```python
from build123d import *

# Parameters (mm, degrees)
SKETCH1_R           = 6
BOSS_EXTRUDE1_DEPTH = 4


with BuildPart() as part:
    # Sketch1 → Boss-Extrude1 (new body)
    with BuildSketch(Plane(origin=(0, 0, 0), x_dir=(1, 0, 0), z_dir=(0, 1, 0))):
        Polygon((9.814954576, 0), (4.907477288, 8.5), (-4.907477288, 8.5), (-9.814954576, 0), (-4.907477288, -8.5), (4.907477288, -8.5), align=None)
        with Locations(Location((0, 0, 0), (0, 0, 270))):
            Circle(SKETCH1_R, mode=Mode.SUBTRACT)
    extrude(amount=BOSS_EXTRUDE1_DEPTH)

    # Sketch2 → Cut-Revolve1 (revolve, cut)
    with BuildSketch(Plane.XY):
        Polygon((-9.814954576, 3.422649731), (-8.814954576, 4), (-9.814954576, 4), align=None)
        Polygon((-9.814954576, 0), (-9.814954576, 0.577350269), (-8.814954576, 0), align=None)
    revolve(axis=Axis((0, 0, 0), (0, 1, 0)), mode=Mode.SUBTRACT)


solid = part.part
```
CAD build for the part. Positions are in the model's coordinates, mm. Round coordinates to 2 decimals unless told otherwise and drop trailing zeros. Order: outer loops, then holes, each group sorted by start corner. A loop starts at its lowest first (then second) coordinate and runs counter-clockwise, first axis right, second up. Notation, with made-up numbers: (-40, 57.25) - (1, 57.25) arc R23 cw to (1, 85.25) - close; hole circle Ø6 at (-2.75, 75.25). An arc over 180 degrees is marked (long way). Answer in a Markdown table with one row per item. Add a question column.
(1) Drop a flat-ended pin along its axis: pin 1 Ø1.5 at (x, y) = (-7.5, 2) entering from +Z. Give the stop position or say it passes through.
(2) Probe L1, parallel to X at y = 2.1, z = 2; L2, parallel to X at y = 0.8, z = -5.5; L3, parallel to Z at x = -2, y = 1.95. List the from-to ranges inside material, lowest first. Write a range as [from, to].
(3) Band-saw the part on D-D on x = -6.75. List the corners of the cut face in (y, z), and give its area (3 significant figures).
(4) Mould opens along X. For faces 1 (the face through (-4.515, 0.156, -7.885)), 2 (the face through (1.802, 1.972, 5.723)), 3 (the face through (-2, 4, -6)) say: +X half, -X half, draft (parallel to the pull), parting line (faces both ways), or undercut.
(5) Band-saw the part on C-C on z = -5.25. List the corners of the cut face in (x, y), and give its area (3 significant figures).
(6) Band-saw the part on B-B on y = 1. List the corners of the cut face in (x, z).
(7) Band-saw the part on A-A on x = 0. List the corners of the cut face in (y, z), and give its area (3 significant figures).
Data:
| question | item | result |
|---|---|---|
| 1 | pin 1 | stops at z = 5.31 |
| 2 | L1 | x = [-8.66, -5.66], [5.66, 8.66] |
| 2 | L2 | x = [-6.64, -2.4], [2.4, 6.64] |
| 2 | L3 | z = [-8.5, -5.66], [5.66, 8.5] |
| 3 | outline | (0, -5.31) - (4, -5.31) - (4, 5.31) - (0, 5.31) - close |
| 3 | area | 42.5 mm^2 |
| 4 | face 1 | -X half |
| 4 | face 2 | undercut |
| 4 | face 3 | draft |
| 5 | outline | (-6.78, 0) - (-2.9, 0) - (-2.9, 4) - (-6.78, 4) - close; (2.9, 0) - (6.78, 0) - (6.78, 4) - (2.9, 4) - close |
| 5 | area | 31.0 mm^2 |
| 6 | outline | (-9.81, 0) - (-4.91, -8.5) - (4.91, -8.5) - (9.81, 0) - (4.91, 8.5) - (-4.91, 8.5) - close; hole circle Ø12 at (0, 0) |
| 7 | outline | (0, -8.5) - (4, -8.5) - (4, -6) - (0, -6) - close; (0, 6) - (4, 6) - (4, 8.5) - (0, 8.5) - close |
| 7 | area | 20.0 mm^2 |
